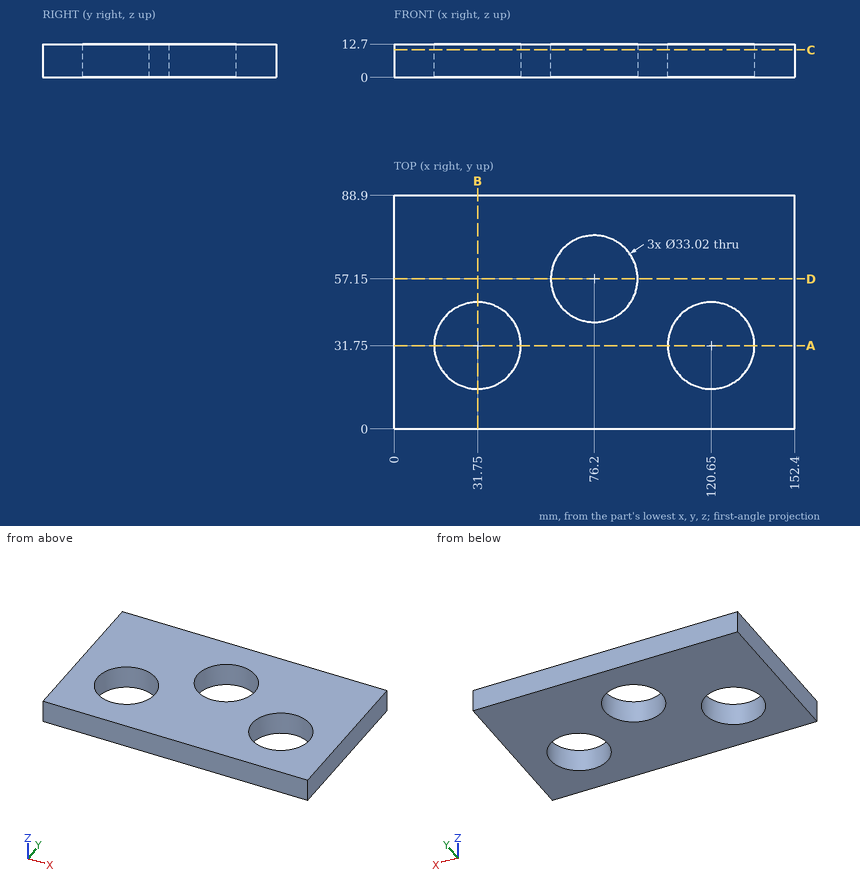
Geometry: see drawing. Coordinates: mm, zero at the bounding-box minimum. Give positions to 0.01 mm unless a question says otherwise; leave off trailing zeros. Write each loop counter-clockwise with the first axis right and the second up, starting at its lowest first coordinate (ties: lowest second). Pieces come first, ordered by that corner, then holes. Notation, with made-up numbers: (77.25, 68) - (93.25, 68) arc R7 cw to (93.25, 73) - close; hole circle Ø1 at (12.5, 29.5). An arc over 180 degrees is marked (long way). Return JSON: item names as keys, results as strings. Group by question number.
1) Line query: line 1 (Y direction, x = 77, z = 4); line 2 (Y direction, x = 120.65, z = 9.25); line 3 (X direction, y = 34, z = 3.5). Output: solid intervals per line, ascending.
2) Section C-C on z = 10.5. Return the cut outline in (x, y), plus the area to 3 significant figures.
3) Section A-A on y = 31.75. Return the cut outline in (x, z), plus the area to 3 significant figures.
4) Section D-D on y = 57.15. Return the cut outline in (x, z), plus the area to 3 significant figures.
5) First-contact query: P1, Ø6, axis at x = 136, y = 27.5, coming from the -Z side. Flat tip, straight axial feed; report the tip coordinate or a pass-through.
6) Section B-B on x = 31.75. Return the cut outline in (y, z), plus the area to 3 significant figures.
Filled in:
{
 "1": {"line 1": "y = 0 to 40.66, 73.64 to 88.9", "line 2": "y = 0 to 15.24, 48.26 to 88.9", "line 3": "x = 0 to 15.39, 48.11 to 104.29, 137.01 to 152.4"},
 "2": {"outline": "(0, 0) - (152.4, 0) - (152.4, 88.9) - (0, 88.9) - close; hole circle Ø33.02 at (31.75, 31.75); hole circle Ø33.02 at (76.2, 57.15); hole circle Ø33.02 at (120.65, 31.75)", "area": "11,000 mm^2"},
 "3": {"outline": "(0, 0) - (15.24, 0) - (15.24, 12.7) - (0, 12.7) - close; (48.26, 0) - (104.14, 0) - (104.14, 12.7) - (48.26, 12.7) - close; (137.16, 0) - (152.4, 0) - (152.4, 12.7) - (137.16, 12.7) - close", "area": "1,100 mm^2"},
 "4": {"outline": "(0, 0) - (59.69, 0) - (59.69, 12.7) - (0, 12.7) - close; (92.71, 0) - (152.4, 0) - (152.4, 12.7) - (92.71, 12.7) - close", "area": "1,520 mm^2"},
 "5": {"P1": "stops at z = 0"},
 "6": {"outline": "(0, 0) - (15.24, 0) - (15.24, 12.7) - (0, 12.7) - close; (48.26, 0) - (88.9, 0) - (88.9, 12.7) - (48.26, 12.7) - close", "area": "710 mm^2"}
}
